Here's how the part is built. I have some questions about the finished solid (model axes, mm). A direction names the side the tool comes from. Coordinates: 2 decimals unless noted, no trailing zeros. Order: outer loops, then holes, each group sorted by start corner. A loop starts at its lowest first (then second) coordinate and runs counter-clockwise, first axis right, second up. Notation, with made-up numbers: M 35,-37.5 L 46,-37.5 A12 cw 46,-28.5 Z; hole C 48,11.25 d6. An arc over 180 degrees is marked long. One line per question, with ' | ' between items. Start each with the question number.
```python
from build123d import *

# Parameters (mm, degrees)
BOSS_EXTRUDE3_DEPTH     = 10
SKETCH5_W               = 30
SKETCH5_H               = 25
BOSS_EXTRUDE5_DEPTH     = 5
BOSS_EXTRUDE7_DEPTH     = 5
BOSS_EXTRUDE8_DEPTH     = 71
BOSS_EXTRUDE9_DEPTH     = 125
SKETCH12_R              = 3.25
CUT_EXTRUDE1_DEPTH      = 6
CUT_EXTRUDE1_DEPTH_BACK = 15
SKETCH13_R              = 1.75
CUT_EXTRUDE2_DEPTH      = 5
CUT_EXTRUDE2_DEPTH_BACK = 15
SKETCH14_R              = 3.5
CUT_EXTRUDE3_DEPTH      = 10
SKETCH15_R              = 3.5
CUT_EXTRUDE4_DEPTH      = 10


with BuildPart() as part:
    # Sketch3 → Boss-Extrude3 (new body)
    with BuildSketch(Plane.XY):
        Polygon((0, 0), (0, -5), (20, -5), (20, -25), (30, -25), (30, 22.02), (20, 22.02), (20, 0), align=None)
    extrude(amount=BOSS_EXTRUDE3_DEPTH)

    # Sketch5 → Boss-Extrude5 (add)
    with BuildSketch(Plane.XY.offset(10)):
        with Locations((15, -12.5)):
            Rectangle(SKETCH5_W, SKETCH5_H)
    extrude(amount=BOSS_EXTRUDE5_DEPTH)

    # Sketch7 → Boss-Extrude7 (add)
    with BuildSketch(Plane(origin=(0, 0, 0), x_dir=(-1, 0, 0), z_dir=(0, 0, -1))):
        Polygon((0, 0), (-20, 0), (-20.758888401, 0), (-30, 0), (-30, -25), (-20, -25), (-20, -5), (0, -5), align=None)
    extrude(amount=BOSS_EXTRUDE7_DEPTH)

    # Sketch10 → Boss-Extrude8 (add)
    with BuildSketch(Plane.XZ.offset(25)):
        Polygon((0, 10), (20, 10), (20, -5), (30, -5), (30, 15), (0, 15), align=None)
    extrude(amount=BOSS_EXTRUDE8_DEPTH)

    # Sketch11 → Boss-Extrude9 (add)
    with BuildSketch(Plane.ZY):
        Polygon((10, 0), (-5, 0), (-5, -5), (10, -5), (10, -9.348527433), (15, -9.348527433), (15, -5), (15, 0), align=None)
    extrude(amount=BOSS_EXTRUDE9_DEPTH)

    # Sketch12 → Cut-Extrude1 (cut, two sides)
    with BuildSketch(Plane.XY.offset(15)) as cut_extrude1_sk:
        with Locations((9, -13)):
            Circle(SKETCH12_R)
    extrude(amount=CUT_EXTRUDE1_DEPTH, mode=Mode.SUBTRACT)
    extrude(cut_extrude1_sk.sketch, amount=-CUT_EXTRUDE1_DEPTH_BACK, mode=Mode.SUBTRACT)

    # Sketch13 → Cut-Extrude2 (cut, two sides)
    with BuildSketch(Plane(origin=(0, 0, 0), x_dir=(1, 0, 0), z_dir=(0, 1, 0))) as cut_extrude2_sk:
        with Locations((-52.5, -5.597603222)):
            Circle(SKETCH13_R)
    extrude(amount=CUT_EXTRUDE2_DEPTH, mode=Mode.SUBTRACT)
    extrude(cut_extrude2_sk.sketch, amount=-CUT_EXTRUDE2_DEPTH_BACK, mode=Mode.SUBTRACT)

    # Sketch14 → Cut-Extrude3 (cut)
    with BuildSketch(Plane(origin=(0, 0, 0), x_dir=(1, 0, 0), z_dir=(0, 1, 0))):
        with Locations((-102, -2)):
            Circle(SKETCH14_R)
    extrude(amount=-CUT_EXTRUDE3_DEPTH, mode=Mode.SUBTRACT)

    # Sketch15 → Cut-Extrude4 (cut)
    with BuildSketch(Plane(origin=(0, 0, 0), x_dir=(1, 0, 0), z_dir=(0, 1, 0))):
        with Locations((9, -2)):
            Circle(SKETCH15_R)
    extrude(amount=-CUT_EXTRUDE4_DEPTH, mode=Mode.SUBTRACT)


solid = part.part
```
1. Will these pins go through, and if not, where does the flat tip stop? pin 1 (4 mm diameter, centred on x = 5, y = -55.5, fed in from -Z); pin 2 (2.5 mm diameter, centred on x = -73.5, z = 13, fed in from -Y); pin 3 (12 mm diameter, centred on y = -64, z = 2.5, fed in from -X).
2. Imagine slicing it at D-D (x = -52.5). List the corners of the cut face in (y, z) for me, then the cut area to 3 significant figures.
3. I need wall thicknesses on line 1 (X direction, y = -3, z = 2); line 2 (Y direction, x = 9, z = 11.3); line 3 (Y direction, x = -102.5, z = 12). Which ranges of each line are inside material? Lowest first, please.
4. We'd pull the mould along Z, two halves only. Please class faces 1 (the face through (5.503, -2.465, 1.846)), 2 (the face through (-62, -9.349, 12)), 3 (the face through (2, -44, 10)): released by +Z, released by -Z, zero draft, split by the parting line, or undercut.
5. Imagine slicing it at A-A (y = -13). List the corners of the cut face in (x, z) for me.
6. Imagine slicing it at B-B (x = 9). List the corners of the cut face in (y, z) for me.
7. Which directions (+Z, -Z, +X, -X, +Y, -Y) give clear straight access to the entire face, cutting with the end or side of a thin tool? Please do faces 4 (the face through (20, -50, 3)), 5 (the face through (25, 11, 10)), 6 (the face through (25, 11, 0)).
8. Imagine slicing it at C-C (z = 2). List the corners of the cut face in (x, y) for me.
Entries:
1) pin 1: z = 10 | pin 2: y = -9.35 | pin 3: x = 20
2) outline: M -9.35,10 L -5,10 L -5,7.35 L 0,7.35 L 0,15 L -9.35,15 Z; M -5,-5 L 0,-5 L 0,3.85 L -5,3.85 Z | area: 104 mm²
3) line 1: -125 to -105.5, -98.5 to 5.5, 12.5 to 30 | line 2: -96 to -16.25, -9.75 to 0 | line 3: -9.35 to 0
4) face 1: undercut | face 2: zero draft | face 3: released by -Z
5) outline: M 0,10 L 5.75,10 L 5.75,15 L 0,15 Z; M 12.25,10 L 20,10 L 20,-5 L 30,-5 L 30,15 L 12.25,15 Z
6) outline: M -96,10 L -16.25,10 L -16.25,15 L -96,15 Z; M -9.75,10 L -5,10 L -5,5.5 L 0,5.5 L 0,15 L -9.75,15 Z; M -5,-5 L 0,-5 L 0,-1.5 L -5,-1.5 Z
7) face 4: -Z, -X, -Y | face 5: +Z, +X, -X, +Y | face 6: -Z, +X, -X, +Y
8) outline: M -125,-5 L -105.5,-5 L -105.5,0 L -125,0 Z; M -98.5,-5 L 5.5,-5 L 5.5,0 L -98.5,0 Z; M 12.5,-5 L 20,-5 L 20,-96 L 30,-96 L 30,22.02 L 20,22.02 L 20,0 L 12.5,0 Z
